For this review, take the finished solid that the model builds, in its own axes (mm). Give positions to 0.01 mm unless a question says otherwise; leave off trailing zeros. Write each loop counter-clockwise with the first axis right and the second up, starting at its lowest first coordinate (ties: lowest second). Pieces come first, ordered by that corner, then holes. Notation, with made-up numbers: (-32.5, 16.5) -> (-22.5, 16.5) arc R8 ccw to (-22.5, 22.5) -> close; hole circle Ø8 at (86, 26). An arc over 180 degrees is marked (long way). Return JSON: item names as keys, results as strings.
from build123d import *

# Parameters (mm, degrees)
F0_R     = 85
F2_R     = 0.5
F4_R     = 105.9677495378
F5_DEPTH = 1


# Not quite as in the source:
# - a fillet or chamfer that OpenCascade refuses, or shapes differently, is made with other operations: its cross-section is extruded or revolved along the edge and cut away or added


with BuildPart() as f3:
    # F0 (on Top) → F3 section 0
    with BuildSketch(Plane.XY):
        Circle(F0_R)
    # F2 (on offset) → F3 section 1
    with BuildSketch(Plane.XY.offset(1000)):
        Circle(F2_R)
    loft()

    # F4 (on Top) → F5 (join)
    with BuildSketch(Plane.XY):
        Circle(F4_R)
    extrude(amount=F5_DEPTH)

    # F6: fillet of radius 50 on 1 edges, made by hand

    # F6_s1 → F6_t2 (revolve)
    with BuildSketch(Plane.XZ):
        with BuildLine():
            ThreePointArc((105.9677495378, 1), (89.0977776327, 17.4521656578), (81.6365703283, 39.8039014399))
            Line((81.6365703283, 39.8039014399), (84.9155, 1))
            Line((84.9155, 1), (105.9677495378, 1))
        make_face()
    revolve(axis=Axis((0, 0, 1), (0, 0, 1)))


solid = f3.part
1. To check wall thickness, follow probe 1 along Y at (x, z) = (-18, 84); probe 2 along X at (y, z) = (14, 374); probe 3 along X at (y, z) = (-25, 515). State the ranges of each line that lie inside material, in increasing order.
Results found:
{"probe 1": "y = -75.79 to 75.79", "probe 2": "x = -51.53 to 51.53", "probe 3": "x = -33.1 to 33.1"}
2. For pin 1 (1.5 mm diameter, centred on y = 51, z = 206.5, fed in from -X); pin 2 (8 mm diameter, centred on x = -10.5, z = 794.5, fed in from +Y); pin 3 (2 mm diameter, centred on x = -45.5, z = 436, fed in from +Y), all flat-tipped, find the tip position at first contact; note any pin that passes through.
Results found:
{"pin 1": "stops at x = -45.15", "pin 2": "stops at y = 16.68", "pin 3": "stops at y = 18.42"}
3. Add section B-B, the plane z = 928. State the section outline as (x, y) points.
Results found:
{"outline": "circle Ø13.17 at (0, 0)"}
4. Add section A-A, the plane z = 480.5. State the section outline as (x, y) points, plus the area to 3 significant figures.
Results found:
{"outline": "circle Ø88.8 at (0, 0)", "area": "6,190 mm²"}
